from build123d import *

# Parameters (mm, degrees)
PAD_DEPTH       = 17
CHAMFER_SIZE    = 10
CHAMFER001_SIZE = 10
SKETCH001_R     = 5
POCKET_DEPTH    = 12.001
PAD001_DEPTH    = 20
PAD002_DEPTH    = 20
SKETCH004_R     = 6
POCKET001_DEPTH = 90.001


with BuildPart() as part:
    # Sketch → Pad (new body, symmetric)
    with BuildSketch(Plane.XZ):
        Polygon((-57.5, 0), (-17.5, 0), (-17.5, 15), (17.5, 15), (17.5, 0), (57.5, 0), (57.5, 12), (32.5, 12), (32.5, 65), (12.5, 65), (12.5, 27), (-12.5, 27), (-12.5, 65), (-32.5, 65), (-32.5, 12), (-57.5, 12), align=None)
    extrude(amount=PAD_DEPTH, both=True)

    # Chamfer
    chamfer_edges = [part.edges().sort_by_distance(p)[0] for p in [
        (57.5, -17, 6),
    ]]
    chamfer(chamfer_edges, length=CHAMFER_SIZE)

    # Chamfer001
    chamfer001_edges = [part.edges().sort_by_distance(p)[0] for p in [
        (-57.5, -17, 6),
    ]]
    chamfer(chamfer001_edges, length=CHAMFER001_SIZE)

    # Sketch001 → Pocket (cut, through all)
    with BuildSketch(Plane(origin=(0, 0, 12), x_dir=(-1, 0, 0), z_dir=(0, 0, 1))):
        with Locations((45, -5)):
            Circle(SKETCH001_R)
        with Locations((-45, -5)):
            Circle(SKETCH001_R)
    extrude(amount=-POCKET_DEPTH, mode=Mode.SUBTRACT)

    # Sketch002 → Pad001 (new body)
    with BuildSketch(Plane(origin=(32.5, 0, 0), x_dir=(0, 0, 1), z_dir=(1, 0, 0))):
        with BuildLine():
            ThreePointArc((65, -17), (69.405883, 0), (65, 17))
            Line((65, 17), (65, -17))
        make_face()
    extrude(amount=-PAD001_DEPTH)

    # Sketch003 → Pad002 (new body)
    with BuildSketch(Plane(origin=(-32.5, 0, 0), x_dir=(0, 0, -1), z_dir=(-1, 0, 0))):
        with BuildLine():
            ThreePointArc((-65, 17), (-69.405883, 0), (-65, -17))
            Line((-65, 17), (-65, -17))
        make_face()
    extrude(amount=-PAD002_DEPTH)

    # Sketch004 → Pocket001 (cut, through all)
    with BuildSketch(Plane(origin=(32.5, 0, 0), x_dir=(0, 0, 1), z_dir=(1, 0, 0))):
        with Locations((45, 0)):
            Circle(SKETCH004_R)
    extrude(amount=-POCKET001_DEPTH, mode=Mode.SUBTRACT)


solid = part.part
Can you work these out from the model? Positions are in its coordinate system, mm. A direction names the side the tool comes from. Coordinates: 2 decimals unless noted, no trailing zeros. Loops run counter-clockwise (first coordinate to the right, second up) from the corner with the lowest first, then second, coordinate; pieces in that order, holes last. Notation, with made-up numbers: M -36.5,34 L -15.5,34 A26 cw -15.5,67 Z; hole C -16,-4 d2. An arc over 180 degrees is marked long. Return JSON: item names as keys, results as strings. Group by question number.
Item 1: On a 3-axis mill with a long thin cutter (end or side, diameter ignored), from which of +Z, -Z, +X, -X, +Y, -Y can I reach the whole of each face in a straight line? I mean faces 1 (the flat face through (-44.8, -0.2, 12)), 2 (the flat face through (32.5, -4, 40)), 3 (the flat face through (-12.5, 0, 53)), 4 (the flat face through (-1, -17, 26)), 5 (the flat face through (0, 0, 15)). Say none if no direction works.
Item 2: I'm going to push flat-ended pins straight in: pin 1 Ø20 at (x, y) = (3.5, -3) entering from +Z; pin 2 Ø10 at (y, z) = (1.5, 34.5) entering from +X; pin 3 Ø6 at (y, z) = (12.5, 55) entering from -X; pin 4 Ø10 at (x, y) = (-7.5, -1) entering from -Z. Where does each tip first touch, or does it pass through?
Item 3: Imagine slicing it at B-B (x = -45). Please give me the cut outline in (y, z).
Item 4: Imagine slicing it at D-D (z = 45). Please give me the cut outline in (x, y).
Item 5: Thinking about a two-plate mould opening in Z: for faces 6 (the cylindrical face through (23, 0, 39)), 7 (the flat face through (12.5, 0, 53)), 8 (the flat face through (-38, 0, 0)), 9 (the cylindrical face through (-22.64, -0.249, 69.405)), which applies, released by +Z, released by -Z, zero draft, split by the parting line, or undercut?
Item 6: Imagine slicing it at C-C (z = 57.5). Please give me the cut outline in (x, y).
Item 7: Imagine slicing it at A-A (z = 8). Please give me the cut outline in (x, y).
Item 8: If I drill on L1, parallel to X at y = -14, z = 61; L2, parallel to X at y = 1, z = 9; L3, parallel to X at y = 5, z = 4, over which ranges is the centre line in solid material (lowest first)? Write a range as from..to.
Verdict:
{
 "1": {"face 1": "+Z, -X, +Y, -Y", "face 2": "+Z, +X, +Y, -Y", "face 3": "+Z, +Y, -Y", "face 4": "+Z, -Z, +X, -X, -Y", "face 5": "-Z, +Y, -Y"},
 "2": {"pin 1": "stops at z = 69.41", "pin 2": "stops at x = 32.5", "pin 3": "stops at x = -32.5", "pin 4": "stops at z = 15"},
 "3": {"outline": "M -17,0 L 0,0 L 0,12 L -17,12 Z; M 10,0 L 17,0 L 17,12 L 10,12 Z"},
 "4": {"outline": "M -32.5,-17 L -12.5,-17 L -12.5,-6 L -32.5,-6 Z; M -32.5,6 L -12.5,6 L -12.5,17 L -32.5,17 Z; M 12.5,-17 L 32.5,-17 L 32.5,-6 L 12.5,-6 Z; M 12.5,6 L 32.5,6 L 32.5,17 L 12.5,17 Z"},
 "5": {"face 6": "undercut", "face 7": "zero draft", "face 8": "released by -Z", "face 9": "released by +Z"},
 "6": {"outline": "M -32.5,-17 L -12.5,-17 L -12.5,17 L -32.5,17 Z; M 12.5,-17 L 32.5,-17 L 32.5,17 L 12.5,17 Z"},
 "7": {"outline": "M -57.5,-7 L -47.5,-17 L -17.5,-17 L -17.5,17 L -57.5,17 Z; M 17.5,-17 L 47.5,-17 L 57.5,-7 L 57.5,17 L 17.5,17 Z; hole C -45,5 d10; hole C 45,5 d10"},
 "8": {"L1": "x = -32.5..-12.5, 12.5..32.5", "L2": "x = -57.5..-48, -42..-17.5, 17.5..42, 48..57.5", "L3": "x = -57.5..-50, -40..-17.5, 17.5..40, 50..57.5"}
}
